Can you work these out from the model? Positions are in its coordinate system, mm. A direction names the side the tool comes from. Round coordinates to 2 decimals unless told otherwise and drop trailing zeros. Write each loop counter-clockwise with the first axis right and the second up, starting at its lowest first coordinate (ties: lowest second). Pieces come first, ordered by that corner, then holes. Notation, with made-up numbers: M 58,12.25 L 88,12.25 A25 cw 88,40.25 Z; hole C 17.5,46 d3. An arc over 180 degrees is marked long. Answer as a JSON object with one key per item and string values. Group by question number.
1) Suppose I cut it at B-B, the plane x = -6.5. Write out the boundary of the cut face in (y, z).
2) Suppose I cut it at C-C, the plane z = 9.5. Write out the boundary of the cut face in (x, y).
3) Suppose I cut it at A-A, the plane z = 0. Write out the boundary of the cut face in (x, y).
4) I'm going to push flat-ended pins straight in: pin 1 Ø2 at (x, y) = (-1.5, 30.5) entering from -Z; pin 2 Ø4 at (x, z) = (2.35, 6.6) entering from -Y; pin 3 Ø12 at (y, z) = (14, -23) entering from -X. Where does each tip first touch, or does it pass through?
5) Suppose I cut it at D-D, the plane y = 3.5. Write out the boundary of the cut face in (x, z), and give its area (3 significant figures).
6) On a 3-axis mill with a long thin cutter (end or side, diameter ignored), from which of +Z, -Z, +X, -X, +Y, -Y can I reach the whole of each face in a straight line? I mean faces 4 (the flat face through (6, 43, 0)), 5 (the flat face through (-7, 0, -26)). Say none if no direction works.
7) If we mould it in two halves opening along X, with no side actions, what happens to faces 1 (the cylindrical face through (1.561, 45.465, 8.104)), 2 (the flat face through (7, 48, 0)), 3 (the cylindrical face through (-4.101, 23.664, -31.232))? For each: +X half, -X half, draft (parallel to the pull), parting line (faces both ways), or undercut.
8) Please list where these lines run through material, in increasing order: L1, parallel to Z at x = 0, y = 44.9; L2, parallel to X at y = 16.5, z = 0.5. Write a range as [from, to].
from build123d import *

# Parameters (mm, degrees)
SKETCH4_R                = 31.5
BOSS_EXTRUDE2_DEPTH      = 48
SKETCH3_R                = 26.5
CUT_EXTRUDE1_DEPTH       = 43
M3_CLEARANCE_HOLE1_D     = 3.4
M3_CLEARANCE_HOLE1_DEPTH = 50
M3_CLEARANCE_HOLE1_TIP   = 1.021463052
SKETCH10_R               = 1.2
CUT_EXTRUDE2_DEPTH       = 10


with BuildPart() as part:
    # Sketch4 → Boss-Extrude2 (new body)
    with BuildSketch(Plane(origin=(0, 0, 0), x_dir=(1, 0, 0), z_dir=(0, 1, 0))):
        Circle(SKETCH4_R)
    extrude(amount=BOSS_EXTRUDE2_DEPTH)

    # Sketch3 → Cut-Extrude1 (cut)
    with BuildSketch(Plane(origin=(0, 0, 0), x_dir=(1, 0, 0), z_dir=(0, 1, 0))):
        Circle(SKETCH3_R)
    extrude(amount=CUT_EXTRUDE1_DEPTH, mode=Mode.SUBTRACT)

    # M3 Clearance Hole1
    with Locations(Plane(origin=(0, 48, 0), x_dir=(1, 0, 0), z_dir=(0, 1, 0))):
        with Locations((-2.345047045, 6.595510166), (2.345047045, -6.595510166)):
            Hole(M3_CLEARANCE_HOLE1_D / 2, depth=M3_CLEARANCE_HOLE1_DEPTH)
            with Locations((0, 0, -(M3_CLEARANCE_HOLE1_DEPTH + M3_CLEARANCE_HOLE1_TIP / 2))):  # 118° drill point
                Cone(0, M3_CLEARANCE_HOLE1_D / 2, M3_CLEARANCE_HOLE1_TIP, mode=Mode.SUBTRACT)

    # Sketch10 → Cut-Extrude2 (cut)
    with BuildSketch(Plane(origin=(0, 48, 0), x_dir=(1, 0, 0), z_dir=(0, 1, 0))):
        Circle(SKETCH10_R)
    extrude(amount=-CUT_EXTRUDE2_DEPTH, mode=Mode.SUBTRACT)


solid = part.part
Results:
{
 "1": {"outline": "M 0,-30.82 L 48,-30.82 L 48,30.82 L 0,30.82 L 0,25.69 L 43,25.69 L 43,-25.69 L 0,-25.69 Z"},
 "2": {"outline": "M -30.03,0 L -24.74,0 L -24.74,43 L 24.74,43 L 24.74,0 L 30.03,0 L 30.03,48 L -30.03,48 Z"},
 "3": {"outline": "M -31.5,0 L -26.5,0 L -26.5,43 L -1.2,43 L -1.2,48 L -31.5,48 Z; M 1.2,43 L 26.5,43 L 26.5,0 L 31.5,0 L 31.5,48 L 1.2,48 Z"},
 "4": {"pin 1": "z = -31.5", "pin 2": "y = 43", "pin 3": "x = -26.52"},
 "5": {"outline": "C 0,0 d63; hole C 0,0 d53", "area": "911 mm^2"},
 "6": {"face 4": "-Y", "face 5": "+Z, -Z, +X, -X, -Y"},
 "7": {"face 1": "undercut", "face 2": "draft", "face 3": "parting line"},
 "8": {"L1": "[-31.5, -1.2], [1.2, 31.5]", "L2": "[-31.5, -26.5], [26.5, 31.5]"}
}
